Verification items for the finished model (mm, model axes). A direction names the side the tool comes from. Coordinates: 2 decimals unless noted, no trailing zeros. Loops run counter-clockwise (first coordinate to the right, second up) from the corner with the lowest first, then second, coordinate; pieces in that order, holes last.
Q1. Sectioned sample at D-D (y = 18). Enter the section's corners in (x, z), then the cut area to 3 significant figures.
Q2. Mould release check, pull along X, two halves, no side actions. Record for faces 1 (the face through (35, 5, 1)), 2 (the face through (25, 25, 0)), 3 (the face through (2, 47, 1)): +X half, -X half, draft (parallel to the pull), parting line (faces both ways), or undercut.
Q3. Sectioned sample at C-C (x = 33). Enter the section's corners in (y, z), then the cut area to 3 significant figures.
Q4. Sectioned sample at B-B (z = 0.4). Enter the section's corners in (x, y).
Q5. Material ranges on probe 1 along X at (y, z) = (5, 1.2); probe 2 along X at (y, z) = (2.5, 0.8); probe 3 along Y at (x, z) = (24.5, 0.85), recorded low to high.
Q6. Sectioned sample at A-A (y = 6). Enter the section's corners in (x, z), then the cut area to 3 significant figures.
Q7. Access from +Z, -Z, +X, -X, +Y, -Y to the whole of each face (thin tool, end or side, straight path). Record for faces 4 (the face through (48, 3, 1)), 5 (the face through (15, 5, 1)).
```python
from build123d import *

# Parameters (mm, degrees)
BOARD_DEPTH = 1.599999


with BuildPart() as part:
    # 草圖1 → Board (new body)
    with BuildSketch(Plane.XY):
        with BuildLine():
            Line((14.99999794, 9.99999778), (14.99999794, 0))
            Line((14.99999794, 0), (4.99999762, 0))
            Line((4.99999762, 0), (0, 4.99999762))
            Line((0, 4.99999762), (0, 44.9999989))
            Line((0, 44.9999989), (4.99999762, 49.99999906))
            Line((4.99999762, 49.99999906), (44.9999989, 49.99999906))
            Line((44.9999989, 49.99999906), (49.99999906, 44.9999989))
            Line((49.99999906, 44.9999989), (49.99999906, 4.99999762))
            Line((49.99999906, 4.99999762), (44.9999989, 0))
            Line((44.9999989, 0), (34.99999858, 0))
            Line((34.99999858, 0), (34.99999604, 9.99999778))
            ThreePointArc((34.99999604, 9.99999778), (24.99999699, 19.99999683), (14.99999794, 9.99999778))
        make_face()
    extrude(amount=BOARD_DEPTH)


solid = part.part
```
Geometry check:
1. outline: (0, 0) - (19, 0) - (19, 1.6) - (0, 1.6) - close; (31, 0) - (50, 0) - (50, 1.6) - (31, 1.6) - close
1. area: 60.8 mm2
2. face 1: undercut
2. face 2: draft
2. face 3: -X half
3. outline: (16, 0) - (50, 0) - (50, 1.6) - (16, 1.6) - close
3. area: 54.4 mm2
4. outline: (0, 5) - (5, 0) - (15, 0) - (15, 10) arc R10 cw to (35, 10) - (35, 0) - (45, 0) - (50, 5) - (50, 45) - (45, 50) - (5, 50) - (0, 45) - close
5. probe 1: x = 0 to 15, 35 to 50
5. probe 2: x = 2.5 to 15, 35 to 47.5
5. probe 3: y = 19.99 to 50
6. outline: (0, 0) - (15, 0) - (15, 1.6) - (0, 1.6) - close; (35, 0) - (50, 0) - (50, 1.6) - (35, 1.6) - close
6. area: 48.0 mm2
7. face 4: +Z, -Z, +X, -Y
7. face 5: +Z, -Z, -Y
